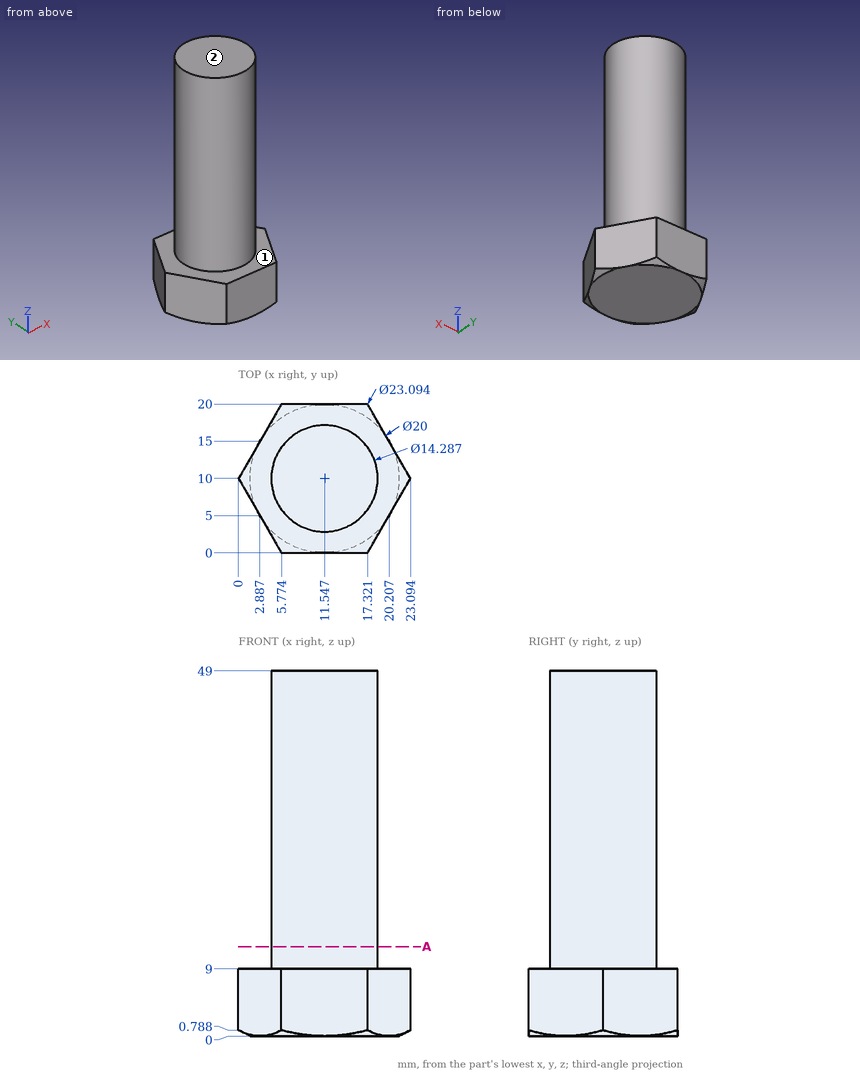
Can you work these out from the drawing? Everything is in mm from the part's minimum corner. A direction names the side the tool comes from. Give positions to 0.01 mm unless a question says otherwise; leave off trailing zeros. Order: outer loops, then holes, each group sorted by start corner. A loop starts at its lowest first (then second) coordinate and runs counter-clockwise, first axis right, second up. Notation, with made-up numbers: (-17.5, 48.5) -> (33.5, 48.5) arc R22 cw to (33.5, 78.5) -> close; hole circle Ø5 at (34.25, -33.75). An arc over 180 degrees is marked (long way). Return JSON: item names as keys, results as strings.
1. Imagine slicing it at A-A on z = 12. List the corners of the cut face in (x, y) for me, then the cut area to 3 significant figures.
Answer list:
{"outline": "circle Ø14.29 at (11.55, 10)", "area": "160 mm2"}
2. I need wall thicknesses on line 1 (Z direction, x = 2, y = 8); line 2 (X direction, y = 5.5, z = 46) (1 decimal); line 3 (Y direction, x = 13.5, z = 31.5). Which ranges of each line are inside material? Lowest first, please. Write a range as from..to.
Answer list:
{"line 1": "z = 0..9", "line 2": "x = 6..17.1", "line 3": "y = 3.13..16.87"}
3. For pin 1 Ø6 at (y, z) = (8.5, 26.5) entering from +X; pin 2 Ø5 at (x, z) = (15.5, 42) entering from +Y (1 decimal); pin 3 Ø6 at (x, z) = (18, 13) entering from -Y (1 decimal), each with a flat end and sliding along its axis, tell me the tip position at first contact or that it passes through.
Answer list:
{"pin 1": "stops at x = 18.69", "pin 2": "stops at y = 17", "pin 3": "stops at y = 3.7"}
4. On a 3-axis mill with a long thin cutter (end or side, diameter ignored), from which of +Z, -Z, +X, -X, +Y, -Y can I reach the whole of each face in a straight line? I mean the marked faces 1 and 2. Say none if no direction works.
Answer list:
{"face 1": "+Z", "face 2": "+Z, +X, -X, +Y, -Y"}
